Autodesk Inventor part; units mm, degrees
ref_plane "Work Plane1" through (0, 0, 28.2) normal (0, 0, 1) x (1, 0, 0)
ref_plane "YZ Plane" through (0, 0, 0) normal (1, 0, 0) x (0, 1, 0)
ref_plane "XZ Plane" through (0, 0, 0) normal (0, 1, 0) x (-1, 0, 0)
sketch "Sketch1" plane through (0, 0, 0) normal (0, 0, 1) x (1, 0, 0)
  line L0 (0, 0) -> (12, 0)
  line L1 (12, 0) -> (12, 10)
  line L2 (12, 10) -> (0, 10)
  line L3 (0, 10) -> (0, 0)
  dimension "d0" = 10
  dimension "d1" = 12
extrude "Extrusion1" add sketch "Sketch1" along normal blind 20
sketch "Sketch2" plane through (0, 0, 20) normal (0, 0, 1) x (1, 0, 0)
  line L0 (12, 0) -> (12, 10)
  line L1 (0, 0) -> (12, 0)
  line L2 (12, 0) -> (12, 10)
  line L3 (12, 10) -> (0, 10)
  line L4 (0, 10) -> (0, 0)
extrude "Extrusion2" add sketch "Sketch2" along normal blind 9
sketch "Sketch3" plane through (0, 0, 29) normal (0, 0, 1) x (1, 0, 0)
  line L0 (12, 10) -> (0, 10)
  line L1 (0, 10) -> (0, 0)
  line L2 (12, 0) -> (12, 10)
  point P0 (1.5, 5)
  point P1 (10.5, 5)
  dimension "d6" = 5
  dimension "d7" = 5
  dimension "d8" = 9
  dimension "d9" = 1.5
  dimension "d10" = 1.5
hole "Hole1" at (1.5, 5, 29) at (10.5, 5, 29) direction (0, 0, -1) diameter 1.221 depth 0.8
ref_plane "Work Plane1" through (0, 0, 28.2) normal (0, 0, 1) x (1, 0, 0)
sketch "Sketch4" plane through (0, 0, 28.2) normal (0, 0, 1) x (1, 0, 0)
  line L0 (0, 10) -> (0, 0)
  line L1 (12, 0) -> (12, 10)
  line L2 (0, 0) -> (12, 0)
  line L3 (12, 0) -> (12, 10)
  line L4 (12, 10) -> (0, 10)
  line L5 (0, 10) -> (0, 0)
  line L6 (3, 2) -> (9, 2)
  line L7 (9, 2) -> (9, 8)
  line L8 (9, 8) -> (3, 8)
  line L9 (3, 8) -> (3, 2)
  circle A0 centre (10.5, 5) radius 0.6105
  circle A1 centre (1.5, 5) radius 0.6105
  point P0 (6, 5)
  dimension "d19" = 2
  dimension "d20" = 2
  dimension "d21" = 1.5
  dimension "d22" = 1.5
extrude "Extrusion3" cut sketch "Sketch4" against normal blind 8.2 contours L4 L1 L2 L0 | A0 | A1
sketch "Sketch5" plane through (0, 0, 28.2) normal (0, 0, 1) x (1, 0, 0)
  line L0 (12, 10) -> (0, 10)
  line L1 (0, 10) -> (0, 0)
  line L2 (12, 0) -> (12, 10)
  line L3 (0, 0) -> (12, 0)
  circle A0 centre (1.6, 8.4) radius 1.5
  circle A1 centre (10.4, 1.6) radius 1.5
  dimension "d25" = 1.6
  dimension "d26" = 1.6
  dimension "d27" = 1.6
  dimension "d28" = 1.6
  dimension "d29" = 3
extrude "Extrusion4" add sketch "Sketch5" against normal up to surface (8.2 mm away) contours A0 | A1
sketch "Sketch6" plane through (0, 0, 29) normal (0, 0, 1) x (1, 0, 0)
  line L0 (12, 10) -> (0, 10)
  line L1 (0, 0) -> (12, 0)
  line L2 (12, 0) -> (12, 10)
  line L3 (0, 10) -> (0, 0)
  circle A0 centre (6, 5) radius 2
  dimension "d32" = 5
  dimension "d33" = 5
  dimension "d34" = 6
  dimension "d35" = 6
  dimension "d36" = 4
extrude "Extrusion5" add sketch "Sketch6" along normal blind 1 contours A0
sketch "Sketch7" plane through (6, 5, 30) normal (0, 0, 1) x (1, 0, 0)
  circle A0 centre (0, -0.0104) radius 1.5
  line L0 (-1.118, 0.9896) -> (1.118, 0.9896)
  point P0 (-6, -5)
  point P1 (0, -1.5104)
  dimension "d39" = 3
  dimension "d40" = 2.5
extrude "Extrusion6" add sketch "Sketch7" along normal blind 9 contours A0 L0 picked at (0.0594, 0.1598)
chamfer "Chamfer1" distance 0.3 angle 45 1 edges at (6, 3.4896, 39)
sketch "Sketch8" plane through (0, 0, 0) normal (0, 0, -1) x (-1, 0, 0)
  line L0 (-12, 10) -> (0, 10)
  line L1 (-12, 0) -> (-12, 10)
  circle A0 centre (-6, 5) radius 6
  line L2 (-12, 10) -> (-12, 0)
  line L3 (0, 0) -> (-12, 0)
  line L4 (-12, 0) -> (-12, 10)
  line L5 (-12, 10) -> (0, 10)
  line L6 (0, 10) -> (0, 0)
  point P0 (0, 5)
  point P1 (0, 10)
  point P2 (-2.6834, 10)
  point P3 (-2.6834, 0)
  point P4 (-9.3166, 0)
  point P5 (-12, 5)
  point P6 (-9.3166, 10)
  dimension "d46" = 5
  dimension "d47" = 6
extrude "Extrusion7" cut sketch "Sketch8" against normal blind 19.2 contours L0 A0 L1 | A0 L3 L1 | L0 L6 A0 | L6 L3 A0
sketch "Sketch9" plane through (0, 0, 0) normal (0, 0, -1) x (-1, 0, 0)
  arc A0 (-9.3166, 10) -> (-9.3166, 0) centre (-6, 5) ccw
  line L0 (-12, 5) -> (-12, 10)
  line L1 (0, 5) -> (0, 0)
  line L2 (-9.3, 4.25) -> (-9.6, 4.25)
  line L3 (-9.6, 4.25) -> (-9.6, 5.75)
  line L4 (-9.6, 5.75) -> (-9.3, 5.75)
  line L5 (-9.3, 5.75) -> (-9.3, 4.25)
  line L6 (-9.3, 4.25) -> (-9.6, 5.75) construction
  line L7 (-9.6, 4.25) -> (-9.3, 5.75) construction
  line L8 (-2.7, 4.25) -> (-2.4, 4.25)
  line L9 (-2.4, 4.25) -> (-2.4, 5.75)
  line L10 (-2.4, 5.75) -> (-2.7, 5.75)
  line L11 (-2.7, 5.75) -> (-2.7, 4.25)
  line L12 (-2.7, 4.25) -> (-2.4, 5.75) construction
  line L13 (-2.4, 4.25) -> (-2.7, 5.75) construction
  point P0 (-9.45, 5)
  point P1 (-2.55, 5)
  dimension "d50" = 6.9
  dimension "d51" = 0
  dimension "d52" = 0
  dimension "d53" = 2.55
  dimension "d54" = 2.55
  dimension "d55" = 1.5
  dimension "d56" = 0.3
extrude "Extrusion8" add sketch "Sketch9" along normal blind 2
sketch "Sketch10" plane through (0, 0, 0) normal (0, 0, -1) x (-1, 0, 0)
  line L0 (-9.3166, 10) -> (-2.6834, 10)
  line L1 (-12, 0) -> (-12, 5)
  circle A0 centre (-6, 5) radius 2.5
  point P0 (0, 0)
  dimension "d59" = 5
  dimension "d60" = 6
  dimension "d61" = 5
extrude "Extrusion9" add sketch "Sketch10" along normal blind 1.1
equation "\"d20\" = d19"
equation "\"d22\" = d21"
properties part number "N30 gear motor"
Here's how the part is built. I have some questions about the finished solid (model axes, mm). A direction names the side the tool comes from. Round coordinates to 2 decimals unless told otherwise and drop trailing zeros. Order: outer loops, then holes, each group sorted by start corner. A loop starts at its lowest first (then second) coordinate and runs counter-clockwise, first axis right, second up. Notation, with made-up numbers: M 39,-22 L 91,-22 A19 ccw 91,-17 Z; hole C 19,9 d7. An arc over 180 degrees is marked long. Return JSON: item names as keys, results as strings. Group by question number.
1. On a 3-axis mill with a long thin cutter (end or side, diameter ignored), from which of +Z, -Z, +X, -X, +Y, -Y can I reach the whole of each face in a straight line? I mean faces 5 (the face through (6, 5.99, 34)), 6 (the face through (5.9, 8.4, 28.2)), 7 (the face through (4.4, 6.2, 29.5)), 8 (the face through (2.4, 5, -1)). Say none if no direction works.
2. If we section it at D-D on x = 11.5: List the corners of the cut face in (y, z) for me, then the cut area to 3 significant figures.
3. I'm going to push flat-ended pins straight in: pin 1 Ø1.5 at (x, z) = (2, 23) entering from +Y; pin 2 Ø5.5 at (x, y) = (6, 5.5) entering from -Z; pin 3 Ø0.8 at (y, z) = (5, -1) entering from -X. Where does each tip first touch, or does it pass through?
4. If we section it at C-C on y = 8.4: List the corners of the cut face in (x, z) for me, then the cut area to 3 significant figures.
5. If we section it at B-B on z = 10: List the corners of the cut face in (x, y) for me.
6. If we section it at A-A on x = 1.5: List the corners of the cut face in (y, z) for me.
7. If we mould it in two halves opening along Z, with no side actions, what happens to faces 1 (the face through (6.1, 10, 28.6)), 2 (the face through (3, 5, 24)), 3 (the face through (11, 1, 19.2)), 4 (the face through (6, 6.4, 30))? For each: pulls with the +Z half, pulls with the -Z half, needs draft (parallel to the pull), parting line crosses it, or undercut.
8. Please list where these lines run through material, in increasing order: probe 1 along X at (y, z) = (5, 28.8); probe 2 along Z at (x, y) = (10, 3.5); probe 3 along Y at (x, z) = (10.5, 28.8).
Reply:
{
 "1": {"face 5": "+Z, +X, -X, +Y", "face 6": "none", "face 7": "+Z", "face 8": "-Z, -X, +Y, -Y"},
 "2": {"outline": "M 0,19.2 L 2.6,19.2 L 2.6,0 L 7.4,0 L 7.4,19.2 L 10,19.2 L 10,20 L 2.62,20 L 2.62,28.2 L 10,28.2 L 10,29 L 0,29 L 0,28.2 L 0.58,28.2 L 0.58,20 L 0,20 Z", "area": "125 mm^2"},
 "3": {"pin 1": "y = 9.9", "pin 2": "z = -1.1", "pin 3": "x = 2.4"},
 "4": {"outline": "M 0,19.2 L 1.06,19.2 L 1.06,0 L 10.94,0 L 10.94,19.2 L 12,19.2 L 12,20 L 3.1,20 L 3.1,28.2 L 12,28.2 L 12,29 L 0,29 L 0,28.2 L 0.1,28.2 L 0.1,20 L 0,20 Z", "area": "234 mm^2"},
 "5": {"outline": "M 2.68,0 L 9.32,0 A6 ccw 9.32,10 L 2.68,10 A6 ccw Z"},
 "6": {"outline": "M 0,19.2 L 1.03,19.2 L 1.03,0 L 8.97,0 L 8.97,19.2 L 10,19.2 L 10,20 L 9.9,20 L 9.9,28.2 L 10,28.2 L 10,29 L 5.61,29 L 5.61,28.2 L 6.9,28.2 L 6.9,20 L 0,20 Z; M 0,28.2 L 4.39,28.2 L 4.39,29 L 0,29 Z"},
 "7": {"face 1": "needs draft", "face 2": "undercut", "face 3": "pulls with the -Z half", "face 4": "pulls with the +Z half"},
 "8": {"probe 1": "0 to 0.89, 2.11 to 9.89, 11.11 to 12", "probe 2": "0 to 20, 28.2 to 29", "probe 3": "0 to 4.39, 5.61 to 10"}
}
